```python
from build123d import *

# Parameters (mm, degrees)
BOSS_EXTRUDE1_DEPTH = 37
CUT_EXTRUDE1_REACH  = 53.904
FILLET1_R           = 5
CUT_EXTRUDE2_REACH  = 53.904
SKETCH4_R           = 15
SKETCH5_W           = 10
SKETCH5_H           = 8
SKETCH5_R           = 2.25
SKETCH5_R_2         = 1
BOSS_EXTRUDE2_DEPTH = 5
SKETCH5_3_R         = 2.25
SKETCH5_3_R_2       = 1
CUT_EXTRUDE3_DEPTH  = 2


with BuildPart() as part:
    # Sketch1 → Boss-Extrude1 (new body)
    with BuildSketch(Plane(origin=(0, 0, 0), x_dir=(1, 0, 0), z_dir=(0, 1, 0))):
        with BuildLine():
            Line((-25, 0), (25, 0))
            ThreePointArc((25, 0), (32.071067812, -2.928932188), (35, -10))
            Line((35, -10), (-35, -10))
            ThreePointArc((-35, -10), (-32.071067812, -2.928932188), (-25, 0))
        make_face()
    extrude(amount=BOSS_EXTRUDE1_DEPTH)

    # Sketch3 → Cut-Extrude1 (cut, up to next)
    with BuildSketch(Plane.XY.offset(10), mode=Mode.PRIVATE) as cut_extrude1_sk1:
        with BuildLine():
            Line((-30, 37), (-35, 37))
            Line((-35, 37), (-35, 32))
            ThreePointArc((-35, 32), (-33.535533906, 35.535533906), (-30, 37))
        make_face()
    cut_extrude1_tool1 = extrude(cut_extrude1_sk1.sketch, amount=-CUT_EXTRUDE1_REACH, mode=Mode.PRIVATE) & part.part
    # Sketch3 → Cut-Extrude1 (cut, up to next)
    with BuildSketch(Plane.XY.offset(10), mode=Mode.PRIVATE) as cut_extrude1_sk2:
        with BuildLine():
            Line((30, 37), (35, 37))
            Line((35, 37), (35, 32))
            ThreePointArc((35, 32), (33.535533906, 35.535533906), (30, 37))
        make_face()
    cut_extrude1_tool2 = extrude(cut_extrude1_sk2.sketch, amount=-CUT_EXTRUDE1_REACH, mode=Mode.PRIVATE) & part.part
    add(cut_extrude1_tool1.solids().sort_by_distance((-33.88316, 35.88316, 10))[0], mode=Mode.SUBTRACT)
    add(cut_extrude1_tool2.solids().sort_by_distance((33.88316, 35.88316, 10))[0], mode=Mode.SUBTRACT)

    # Fillet1
    # the kernel refuses this fillet: 5 mm, written as the material it takes off along each edge
    with BuildSketch(Plane(origin=(25, 37, 10), x_dir=(0, 0, -1), z_dir=(-1, 0, 0))) as fillet1_piece_1:
        with BuildLine():
            CenterArc((10 - FILLET1_R, FILLET1_R), FILLET1_R, 270, 90)
            Line((10 - FILLET1_R, 0), (10, 0))
            Line((10, 0), (10, FILLET1_R))
        make_face()
    revolve(axis=Axis((25, 37, 10), (0, -1, 0)), revolution_arc=101.622920284, mode=Mode.SUBTRACT)
    with BuildSketch(Plane(origin=(-25, 37, 10), x_dir=(-0.9794947331304567, 0, 0.20146976887288942), z_dir=(0.20146976887288942, 0, 0.9794947331304567))) as fillet1_piece_2:
        with BuildLine():
            CenterArc((10 - FILLET1_R, FILLET1_R), FILLET1_R, 270, 90)
            Line((10, FILLET1_R), (10, 0))
            Line((10, 0), (10 - FILLET1_R, 0))
        make_face()
    revolve(axis=Axis((-25, 37, 10), (0, -1, 0)), revolution_arc=101.622920284, mode=Mode.SUBTRACT)
    with BuildSketch(Plane(origin=(-25, 37, 0), x_dir=(0, 0, 1), z_dir=(1, 0, 0))) as fillet1_piece_3:
        with BuildLine():
            CenterArc((FILLET1_R, FILLET1_R), FILLET1_R, 180, 90)
            Line((0, FILLET1_R), (0, 0))
            Line((0, 0), (FILLET1_R, 0))
        make_face()
    extrude(amount=50, mode=Mode.SUBTRACT)

    # Sketch4 → Cut-Extrude2 (cut, up to next)
    with BuildSketch(Plane.XY.offset(10), mode=Mode.PRIVATE) as cut_extrude2_sk1:
        with Locations((0, 17)):
            Circle(SKETCH4_R)
    cut_extrude2_tool1 = extrude(cut_extrude2_sk1.sketch, amount=-CUT_EXTRUDE2_REACH, mode=Mode.PRIVATE) & part.part
    add(cut_extrude2_tool1.solids().sort_by_distance((0, 17, 10))[0], mode=Mode.SUBTRACT)

    # Sketch5 → Boss-Extrude2 (add)
    # profile 1 of 2: a face of its own
    with BuildSketch(Plane(origin=(-35, 0, 0), x_dir=(0, 0, -1), z_dir=(1, 0, 0))):
        with Locations((-15, 16)):
            Rectangle(SKETCH5_W, SKETCH5_H)
        with Locations((-15, 16)):
            Circle(SKETCH5_R, mode=Mode.SUBTRACT)
    # profile 2 of 2: a face of its own
    with BuildSketch(Plane(origin=(-35, 0, 0), x_dir=(0, 0, -1), z_dir=(1, 0, 0))):
        with Locations((-15, 16)):
            Circle(SKETCH5_R)
        with Locations((-15, 16)):
            Circle(SKETCH5_R_2, mode=Mode.SUBTRACT)
    boss_extrude2 = extrude(amount=BOSS_EXTRUDE2_DEPTH)

    # Sketch5<3> → Cut-Extrude3 (cut)
    with BuildSketch(Plane(origin=(-35, 0, 0), x_dir=(0, 0, -1), z_dir=(1, 0, 0))):
        with Locations((-15, 16)):
            Circle(SKETCH5_3_R)
        with Locations((-15, 16)):
            Circle(SKETCH5_3_R_2, mode=Mode.SUBTRACT)
    cut_extrude3 = extrude(amount=CUT_EXTRUDE3_DEPTH, mode=Mode.SUBTRACT)

    # Mirror1: Boss-Extrude2, Cut-Extrude3 across plane
    add(boss_extrude2.mirror(Plane(origin=(0, 0, 0), x_dir=(0, 0, 1), z_dir=(1, 0, 0))))
    add(cut_extrude3.mirror(Plane(origin=(0, 0, 0), x_dir=(0, 0, 1), z_dir=(1, 0, 0))), mode=Mode.SUBTRACT)


solid = part.part
```
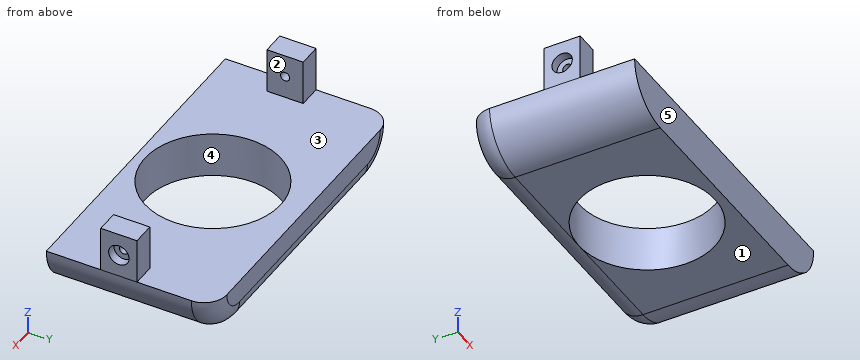
Geometry: final body of the model. Coordinates: model frame, mm. Face numbers are marked on the shaded views. A direction names the side the tool comes from. Round coordinates to 2 decimals unless told otherwise and drop trailing zeros. Order: outer loops, then holes, each group sorted by start corner. A loop starts at its lowest first (then second) coordinate and runs counter-clockwise, first axis right, second up. Notation, with made-up numbers: (54, 52) - (97, 52) arc R20 cw to (97, 88) - close; hole circle Ø2 at (4, 7). An arc over 180 degrees is marked (long way). Write item = value, one per line. Start each with the question number.
Q1. Cut plane B-B on z = 11.25. Return the cut outline in (x, y), and give its area (3 significant figures).
Q2. Ray query, line 1 (Y direction, x = 33.7, z = 15); line 2 (Y direction, x = 0, z = 4.75); line 3 (X direction, y = 17, z = 5.5). Return the intervals inside material, ascending. Write a range as from..to.
Q3. Cut plane D-D on x = -1.5. Return the cut outline in (y, z).
Q4. Pin query (flat end, axial travel): pin 1 (6 mm diameter, centred on x = 21.5, y = 12.5, fed in from +Z); pin 2 (5 mm diameter, centred on y = 5.5, z = 13.5, fed in from -X); pin 3 (2 mm diameter, centred on y = 16.5, z = 15, fed in from +X); pin 4 (4 mm diameter, centred on x = 32.5, z = 14.5, fed in from -Y). Return the tip coordinate at first contact, or that it passes through.
Q5. Pull-direction query (Y, two-part tool) for the marked faces 3, 4 and 5; classes: +Y half, -Y half, draft (parallel to the pull), parting line (faces both ways), or undercut.
Q6. Cut plane C-C on z = 15. Return the cut outline in (x, y).
Q7. Cut plane A-A on y = 26. Return the cut outline in (x, z), and give its area (3 significant figures).
Q8. Access query for the marked faces 1 and 2. Directions: +Z, -Z, +X, -X, +Y, -Y. A direction counts if a zero-diameter tool reaches every point of the face in a straight line with its end or side. Return the directions, or none.
Outcome:
q1.outline = (-35, 12) - (-30, 12) - (-30, 20) - (-35, 20) - close; (30, 12) - (35, 12) - (35, 20) - (30, 20) - close
q1.area = 80.0 mm^2
q2.line_1 = 12..13.75, 18.25..20
q2.line_2 = 0..2, 32..36.99
q2.line_3 = -33.93..-15, 15..33.93
q3.outline = (0, 0) - (2.08, 0) - (2.08, 10) - (0, 10) - close; (31.92, 0) - (32, 0) arc R5 ccw to (37, 5) - (37, 10) - (31.92, 10) - close
q4.pin_1 = 10
q4.pin_2 = through
q4.pin_3 = 33
q4.pin_4 = 12
q5.face_3 = draft
q5.face_4 = undercut
q5.face_5 = -Y half
q6.outline = (-35, 12) - (-30, 12) - (-30, 15) - (-33, 15) - (-33, 13.75) - (-35, 13.75) - close; (-35, 18.25) - (-33, 18.25) - (-33, 17) - (-30, 17) - (-30, 20) - (-35, 20) - close; (30, 12) - (35, 12) - (35, 13.75) - (33, 13.75) - (33, 15) - (30, 15) - close; (30, 17) - (33, 17) - (33, 18.25) - (35, 18.25) - (35, 20) - (30, 20) - close
q7.outline = (-35, 10) arc R10 ccw to (-25, 0) - (-12, 0) - (-12, 10) - close; (12, 0) - (25, 0) arc R10 ccw to (35, 10) - (12, 10) - close
q7.area = 417 mm^2
q8.face_1 = -Z, +X, -X, +Y, -Y
q8.face_2 = +Z, +Y, -Y
